```python
from build123d import *

# Parameters (mm, degrees)
BOSS_EXTRUDE1_DEPTH = 180


with BuildPart() as part:
    # Sketch3 → Boss-Extrude1 (new body)
    with BuildSketch(Plane(origin=(0, 0, 0), x_dir=(0, 0, -1), z_dir=(1, 0, 0))):
        with BuildLine():
            Line((-5.515685425, 6.807463915), (-2.601114729, 3.892893219))
            ThreePointArc((-2.601114729, 3.892893219), (-2.27669138, 3.676120467), (-1.894007948, 3.6))
            Line((-1.894007948, 3.6), (0, 3.6))
            Line((0, 3.6), (0, 2.15))
            ThreePointArc((0, 2.15), (-1.52027958, 1.52027958), (-2.15, 0))
            Line((-2.15, 0), (-3.6, 0))
            Line((-3.6, 0), (-3.6, 1.894007948))
            ThreePointArc((-3.6, 1.894007948), (-3.676120467, 2.27669138), (-3.892893219, 2.601114729))
            Line((-3.892893219, 2.601114729), (-6.807463915, 5.515685425))
            ThreePointArc((-6.807463915, 5.515685425), (-7.679296086, 5.689103626), (-8.17314934, 4.95))
            Line((-8.17314934, 4.95), (-8.17314934, 2.7))
            ThreePointArc((-8.17314934, 2.7), (-8.231727984, 2.558578644), (-8.37314934, 2.5))
            Line((-8.37314934, 2.5), (-9.4, 2.5))
            ThreePointArc((-9.4, 2.5), (-9.824264069, 2.675735931), (-10, 3.1))
            Line((-10, 3.1), (-10, 8.5))
            ThreePointArc((-10, 8.5), (-9.560660172, 9.560660172), (-8.5, 10))
            Line((-8.5, 10), (-3.1, 10))
            ThreePointArc((-3.1, 10), (-2.675735931, 9.824264069), (-2.5, 9.4))
            Line((-2.5, 9.4), (-2.5, 8.37314934))
            ThreePointArc((-2.5, 8.37314934), (-2.558578644, 8.231727984), (-2.7, 8.17314934))
            Line((-2.7, 8.17314934), (-4.95, 8.17314934))
            ThreePointArc((-4.95, 8.17314934), (-5.689103626, 7.679296086), (-5.515685425, 6.807463915))
        make_face()
    extrude(amount=-BOSS_EXTRUDE1_DEPTH)

    # Mirror1: part across plane


with BuildPart() as part_1:
    add(part.part)
    add(part.part.mirror(Plane.ZX))

    # Mirror2: part across plane


with BuildPart() as part_2:
    add(part_1.part)
    add(part_1.part.mirror(Plane.XY))


solid = part_2.part
```
Part model, mm, in its own coordinate system. A direction names the side the tool comes from. Coordinates: 2 decimals unless noted, no trailing zeros. Put each result on its own line as item: value. Start each with the question number.
(1) Pin check, flat tips, straight feed: pin 1 Ø1.9 at (x, y) = (-47.5, -0.5) entering from +Z; pin 2 Ø10 at (y, z) = (-0.5, 4) entering from -X; pin 3 Ø1.9 at (x, z) = (-97.5, 0.5) entering from +Y; pin 4 Ø1.1 at (x, y) = (-45, -0.5) entering from -Z. Stop position of each tip, or through.
(2) Mould opens along Y. For faces 6 (the face through (-89, 6, -10)), 7 (the face through (-88.74, 4.04, -5.33)), 8 (the face through (-89, 3.6, 0)) say: pulls with the +Y half, pulls with the -Y half, needs draft (parallel to the pull), parting line crosses it, or undercut.
(3) Which spindle directions (+Z, -Z, +X, -X, +Y, -Y) get a long thin tool onto all of the face, cutting with end or side? Do faces 1 (the face through (-89, -10, 6)), 2 (the face through (-88.74, -4.04, -5.33)), 3 (the face through (-180, -2.4, 0.1)), 4 (the face through (-89, 0, -3.6)), 5 (the face through (-89, -3.6, 0)). Say none if no direction does.
(4) Probe line 1 along Y through (x, z) = (-152, 6.25); line 2 along Y through (x, z) = (-39, -1); line 3 along Z through (x, y) = (-99, -0.25). List the from-to ranges inside material, lowest first. Write a range as [from, to].
Determined:
1. pin 1: stops at z = 3.6
1. pin 2: stops at x = -180
1. pin 3: stops at y = 3.6
1. pin 4: stops at z = -3.6
2. face 6: needs draft
2. face 7: undercut
2. face 8: pulls with the +Y half
3. face 1: +Z, -Z, +X, -X, -Y
3. face 2: +X, -X
3. face 3: +Z, -Z, -X, +Y, -Y
3. face 4: -Z, +X, -X
3. face 5: +X, -X, -Y
4. line 1: y = [-10, -4.96], [4.96, 10]
4. line 2: y = [-3.6, -1.9], [1.9, 3.6]
4. line 3: z = [-3.6, -2.14], [2.14, 3.6]
